Job drawing, mm, ordinate dimensions from the low corner. One solid piece. A direction names the side the tool comes from. Give positions to 0.01 mm unless a question says otherwise; leave off trailing zeros. Write each loop counter-clockwise with the first axis right and the second up, starting at its lowest first coordinate (ties: lowest second). Pieces come first, ordered by that corner, then holes. Notation, with made-up numbers: (45.25, 32.5) - (53.25, 32.5) arc R13 ccw to (53.25, 42.5) - close; hole circle Ø3 at (78, 7). An arc over 180 degrees is marked (long way). Put each result on its own line as item: value. Start each with the question number.
1. Tool access for the marked faces 1 and 2: list every direction of +Z, -Z, +X, -X, +Y, -Y with a clear straight run to the whole face (end or side of a thin tool).
2. Drop flat-ended pins along their axis: pin 1 (2 mm diameter, centred on x = 32.5, y = 20.5, fed in from +Z); pin 2 (2 mm diameter, centred on x = 26, z = 1, fed in from -Y); pin 3 (0.8 mm diameter, centred on x = 4.5, z = 1, fed in from -Y). Give the stop position or say it passes through.
3. Cut at D-D on z = 1.75. List the corners of the cut face in (x, y) (1 decimal).
4. Cut at B-B on x = 8. List the corners of the cut face in (y, z).
5. Cut at C-C on y = 10.5. List the corners of the cut face in (x, z).
6. Cut at A-A on y = 17. List the corners of the cut face in (x, z).
7. Wall check: line 1 (X direction, y = 13.75, z = 1); line 2 (Z direction, x = 12, y = 8.75); line 3 (Y direction, x = 14.5, z = 2). Give the ranges that are in metal, low to high.
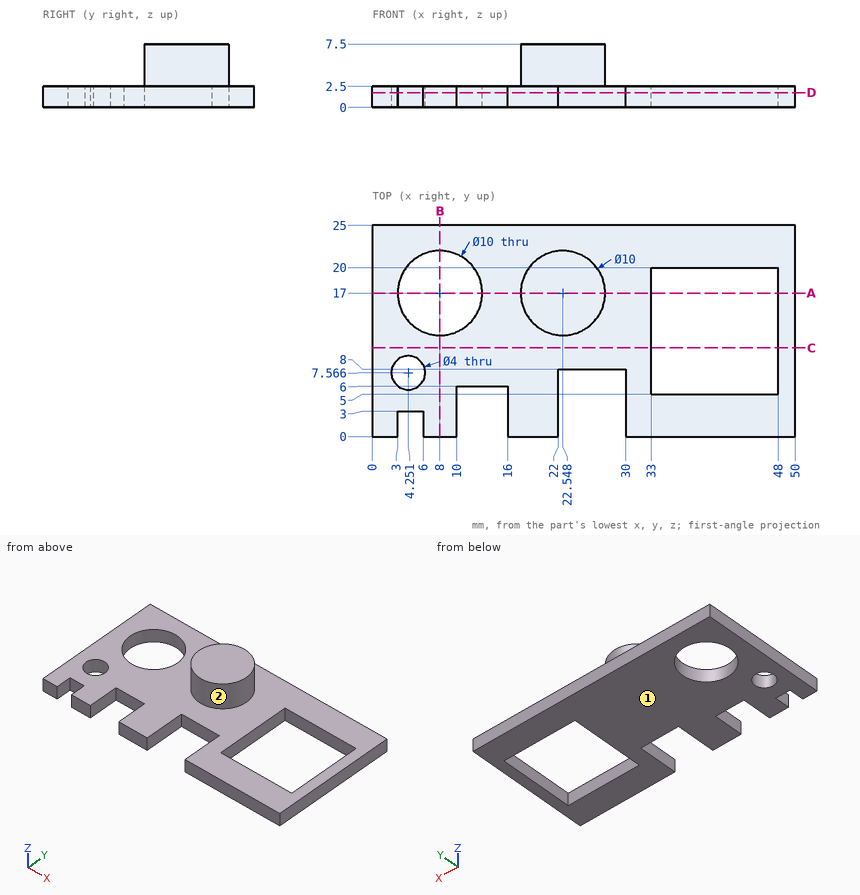
Report:
1. face 1: -Z, +X, -X, +Y, -Y
1. face 2: +Z
2. pin 1: stops at z = 2.5
2. pin 2: stops at y = 8
2. pin 3: stops at y = 3
3. outline: (0, 0) - (3, 0) - (3, 3) - (6, 3) - (6, 0) - (10, 0) - (10, 6) - (16, 6) - (16, 0) - (22, 0) - (22, 8) - (30, 8) - (30, 0) - (50, 0) - (50, 25) - (0, 25) - close; hole circle Ø4 at (4.3, 7.6); hole circle Ø10 at (8, 17); hole (33, 5) - (48, 5) - (48, 20) - (33, 20) - close
4. outline: (0, 0) - (12, 0) - (12, 2.5) - (0, 2.5) - close; (22, 0) - (25, 0) - (25, 2.5) - (22, 2.5) - close
5. outline: (0, 0) - (33, 0) - (33, 2.5) - (0, 2.5) - close; (48, 0) - (50, 0) - (50, 2.5) - (48, 2.5) - close
6. outline: (0, 0) - (3, 0) - (3, 2.5) - (0, 2.5) - close; (13, 0) - (33, 0) - (33, 2.5) - (27.55, 2.5) - (27.55, 7.5) - (17.55, 7.5) - (17.55, 2.5) - (13, 2.5) - close; (48, 0) - (50, 0) - (50, 2.5) - (48, 2.5) - close
7. line 1: x = 0 to 4.2, 11.8 to 33, 48 to 50
7. line 2: z = 0 to 2.5
7. line 3: y = 6 to 25
